Answer from the drawing. Dimensions are ordinates in mm from the lowest x, y and z of the part. A direction names the side the tool comes from. Coordinates: 2 decimals unless noted, no trailing zeros. Loops run counter-clockwise (first coordinate to the right, second up) from the corner with the lowest first, then second, coordinate; pieces in that order, holes last. Notation, with made-up numbers: (17, 20) - (46, 20) arc R27 cw to (46, 45) - close; hole circle Ø11 at (48.25, 0). An arc over 180 degrees is marked (long way). Use one line per item in the form item = value. Start each with the question number.
1) Each of these flat-tipped pins is pushed along its axis until it touches: P1, Ø3, axis at x = 21.5, z = 5.5, coming from the -Y side; P2, Ø5, axis at x = 17, z = 4, coming from the +Y side; P3, Ø3, axis at y = 5.5, z = 7, coming from the +X side; P4, Ø0.5, axis at x = 16.5, y = 3.5, coming from the -Z side. Where does it stop, or does it pass through?
2) The mould has two halves that part along X. Classify the marked faces 4, 5 and 6: released by +X, released by -X, zero draft, split by the parting line, or undercut.
3) A cutting plane is placed at A-A (y = 1). Give the vertices of the cut face in (x, z), and give its area (3 significant figures).
4) A cutting plane is placed at B-B (z = 13.75). Give the vertices of the cut face in (x, y), and give its area (3 significant figures).
5) Consider line 1 (Y direction, x = 25, z = 4.5); line 2 (X direction, y = 5.75, z = 4); line 3 (X direction, y = 0.75, z = 4). Determine where each line is inside the solid, lowest interval first.
6) Which of the six approach directions +Z, -Z, +X, -X, +Y, -Y give full straight-line access (tool end or side, diameter ignored) to the marked faces 1, 2 and 3?
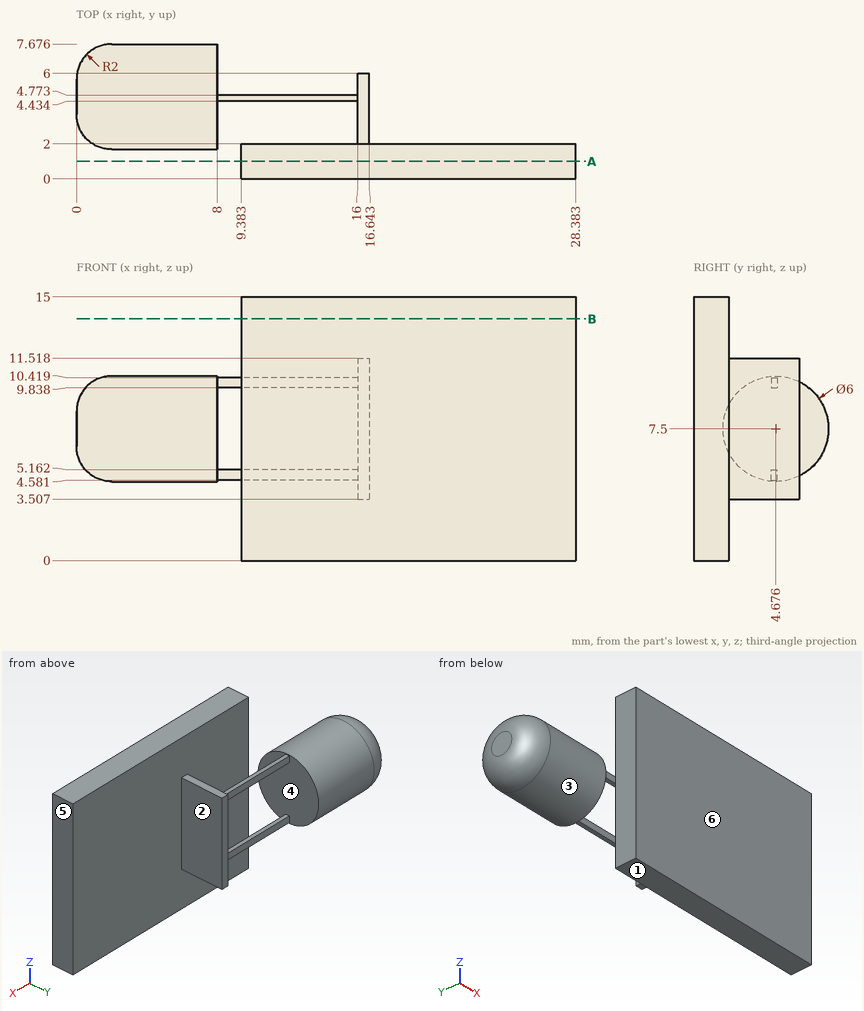
Found:
q1.P1 = 0
q1.P2 = 6
q1.P3 = 16.64
q1.P4 = 3.51
q2.face_4 = undercut
q2.face_5 = released by +X
q2.face_6 = zero draft
q3.outline = (9.38, 0) - (28.38, 0) - (28.38, 15) - (9.38, 15) - close
q3.area = 285 mm^2
q4.outline = (9.38, 0) - (28.38, 0) - (28.38, 2) - (9.38, 2) - close
q4.area = 38.0 mm^2
q5.line_1 = 0 to 2
q5.line_2 = 16 to 16.64
q5.line_3 = 9.38 to 28.38
q6.face_1 = -Z, +X, -X, +Y, -Y
q6.face_2 = +Z, -Z, +X, +Y
q6.face_3 = -X
